```python
from build123d import *

# Parameters (mm, degrees)
F0_W     = 60
F0_H     = 90
F1_DEPTH = 15
F2_W     = 60
F2_H     = 1
F3_DEPTH = 7.5
F4_W     = 13
F4_H     = 1.5
F5_DEPTH = 3
F6_R     = 0.74999
F7_W     = 13
F7_H     = 1.5
F8_DEPTH = 3
F9_R     = 0.74999


# Not quite as in the source:
# - a fillet or chamfer is up to 0.001 mm smaller than in the source, because OpenCascade refuses the exact size


with BuildPart() as f1:
    # F0 (on Top) → F1 (new body)
    with BuildSketch(Plane.XY):
        Rectangle(F0_W, F0_H)
        with BuildLine():
            ThreePointArc((-20, 34.5), (-19.1213203436, 36.6213203436), (-17, 37.5))
            Line((-17, 37.5), (17, 37.5))
            ThreePointArc((17, 37.5), (19.1213203436, 36.6213203436), (20, 34.5))
            Line((20, 34.5), (20, -34.5))
            ThreePointArc((20, -34.5), (19.1213203436, -36.6213203436), (17, -37.5))
            Line((17, -37.5), (-17, -37.5))
            ThreePointArc((-17, -37.5), (-19.1213203436, -36.6213203436), (-20, -34.5))
            Line((-20, -34.5), (-20, 34.5))
        make_face(mode=Mode.SUBTRACT)
    extrude(amount=F1_DEPTH)

    # F2 (on face) → F3 (cut)
    with BuildSketch(Plane.XY.offset(15)):
        with Locations((0, -33.5)):
            Rectangle(F2_W, F2_H)
        with Locations((0, -30)):
            Rectangle(F2_W, F2_H)
        with Locations((0, -26.5)):
            Rectangle(F2_W, F2_H)
        with Locations((0, -23)):
            Rectangle(F2_W, F2_H)
        with Locations((0, -19.5)):
            Rectangle(F2_W, F2_H)
        with Locations((0, -16)):
            Rectangle(F2_W, F2_H)
        with Locations((0, -12.5)):
            Rectangle(F2_W, F2_H)
        with Locations((0, -9)):
            Rectangle(F2_W, F2_H)
        with Locations((0, -5.5)):
            Rectangle(F2_W, F2_H)
        with Locations((0, -2)):
            Rectangle(F2_W, F2_H)
        with Locations((0, 1.5)):
            Rectangle(F2_W, F2_H)
        with Locations((0, 5)):
            Rectangle(F2_W, F2_H)
        with Locations((0, 8.5)):
            Rectangle(F2_W, F2_H)
        with Locations((0, 12)):
            Rectangle(F2_W, F2_H)
        with Locations((0, 15.5)):
            Rectangle(F2_W, F2_H)
        with Locations((0, 19)):
            Rectangle(F2_W, F2_H)
        with Locations((0, 22.5)):
            Rectangle(F2_W, F2_H)
        with Locations((0, 26)):
            Rectangle(F2_W, F2_H)
        with Locations((0, 29.5)):
            Rectangle(F2_W, F2_H)
        with Locations((0, 33)):
            Rectangle(F2_W, F2_H)
    extrude(amount=-F3_DEPTH, mode=Mode.SUBTRACT)

    # F4 (on face) → F5 (cut)
    with BuildSketch(Plane.XZ.offset(45)):
        with Locations((1, 8.25)):
            Rectangle(F4_W, F4_H)
    extrude(amount=-F5_DEPTH, mode=Mode.SUBTRACT)

    # F6 (radius 0.75 in the source; OpenCascade refuses exactly that, so slightly less here)
    f6_edges = [f1.edges().sort_by_distance(p)[0] for p in [
        (-5.5, -43.5, 7.5),
        (-5.5, -43.5, 9),
        (7.5, -43.5, 7.5),
        (7.5, -43.5, 9),
    ]]
    fillet(f6_edges, radius=F6_R)

    # F7 (on face) → F8 (cut)
    with BuildSketch(Plane(origin=(0, 45, 0), x_dir=(-1, 0, 0), z_dir=(0, 1, 0))):
        with Locations((-1, 8.25)):
            Rectangle(F7_W, F7_H)
    extrude(amount=-F8_DEPTH, mode=Mode.SUBTRACT)

    # F9 (radius 0.75 in the source; OpenCascade refuses exactly that, so slightly less here)
    f9_edges = [f1.edges().sort_by_distance(p)[0] for p in [
        (-5.5, 43.5, 7.5),
        (-5.5, 43.5, 9),
        (7.5, 43.5, 9),
        (7.5, 43.5, 7.5),
    ]]
    fillet(f9_edges, radius=F9_R)


solid = f1.part
```
Model file for the job. Use its own axes, mm. A direction names the side the tool comes from. Give positions to 0.01 mm unless a question says otherwise; leave off trailing zeros. Loops run counter-clockwise (first coordinate to the right, second up) from the corner with the lowest first, then second, coordinate; pieces in that order, holes last. Notation, with made-up numbers: (44.25, -35.5) -> (99.25, -35.5) arc R10 cw to (99.25, -25.5) -> close; hole circle Ø11 at (74.25, 83.25). An arc over 180 degrees is marked (long way). Use CSV: the item, a comma, the result in double quotes. Start each with the question number.
1) Slice it at C-C on z = 11.75. Give the number of separate pieces and of enclosed holes in the cut face, plus the area to 3 significant figures.
2) Tool access for faces 3 (the flat face through (0, -37.5, 7)), 4 (the flat face through (25, 32.5, 11)), 5 (the flat face through (-25, 17, 15)): list every direction of +Z, -Z, +X, -X, +Y, -Y with a clear straight run to the whole face (end or side of a thin tool).
3) Flat gauge pin, fed straight in: pin 1 Ø0.8 at (x, y) = (-27, 22.5) entering from +Z. Where does the tip first touch, or does it go through?
4) Mould opens along X. For faces 1 (the flat face through (1, -44, 7.5)), 2 (the flat face through (25, -25, 15)) say: released by +X, released by -X, zero draft, split by the parting line, or undercut.
5) Wall check: line 1 (X direction, y = 16.5, z = 6.75); line 2 (Y direction, x = -9.5, z = 1.25); line 3 (Y direction, x = 19, z = 4.5). Give the ranges that are in metal, low to high.
6) Slice it at A-A on z = 2.5. Give the cut face in (x, y).
7) Slice it at B-B on y = -10.5. Give the cut face in (x, z).
Computed values:
1,separate pieces,"40"
1,enclosed holes,"0"
1,area,"2,010 mm^2"
2,face 3,"+Z, -Z"
2,face 4,"+Z, +X, -X"
2,face 5,"+Z, +X, -X, +Y, -Y"
3,pin 1,"stops at z = 7.5"
4,face 1,"undercut"
4,face 2,"zero draft"
5,line 1,"x = -30 to -20, 20 to 30"
5,line 2,"y = -45 to -37.5, 37.5 to 45"
5,line 3,"y = -45 to -36.74, 36.74 to 45"
6,outline,"(-30, -45) -> (30, -45) -> (30, 45) -> (-30, 45) -> close; hole (-20, -34.5) arc R3 ccw to (-17, -37.5) -> (17, -37.5) arc R3 ccw to (20, -34.5) -> (20, 34.5) arc R3 ccw to (17, 37.5) -> (-17, 37.5) arc R3 ccw to (-20, 34.5) -> close"
7,outline,"(-30, 0) -> (-20, 0) -> (-20, 15) -> (-30, 15) -> close; (20, 0) -> (30, 0) -> (30, 15) -> (20, 15) -> close"
